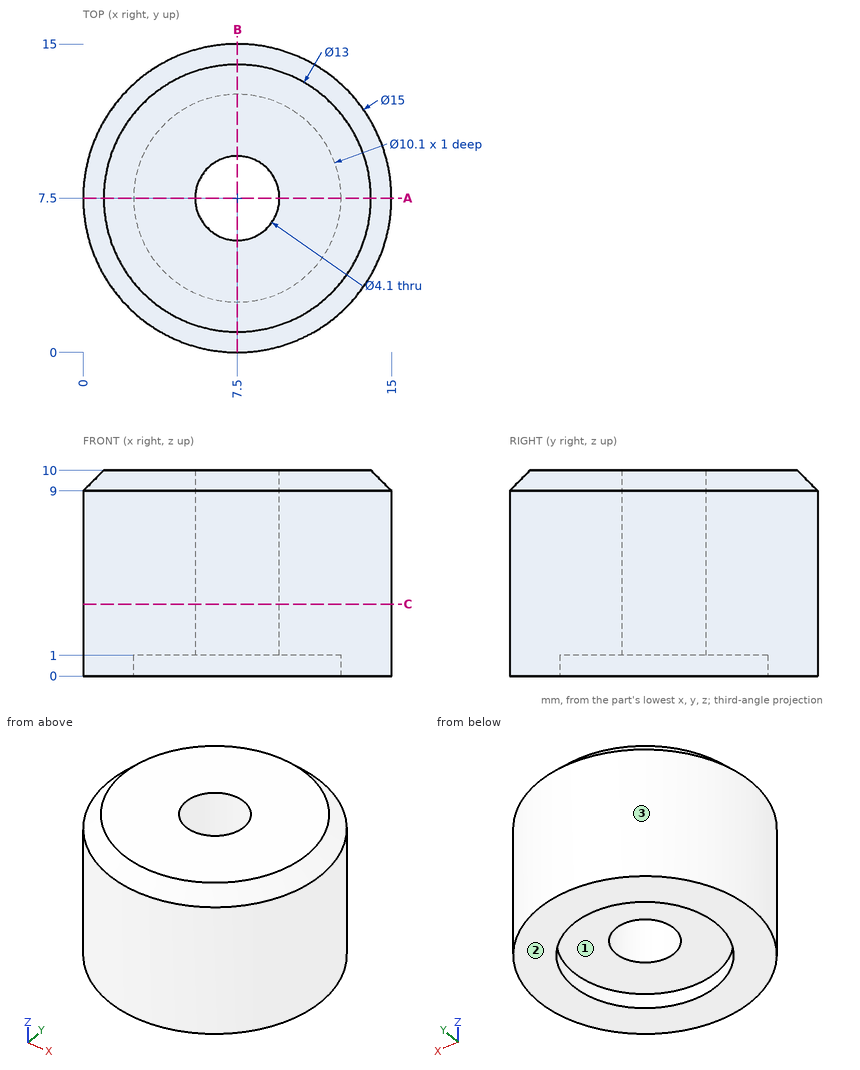
Print and shaded views of the part. All mm, measured from the part's lowest x, y and z. Coordinates: 2 decimals unless noted, no trailing zeros. Write each loop counter-clockwise with the first axis right and the second up, starting at its lowest first coordinate (ties: lowest second). Pieces come first, ordered by that corner, then holes.
(1) Two-plate mould, pull along X, no slides. Class the marked faces 1, 2 and 3: +X half, -X half, draft (parallel to the pull), parting line (faces both ways), or undercut.
(2) Cut at A-A, the plane y = 7.5. List the corners of the cut face in (x, z).
(3) Cut at C-C, the plane z = 3.5. List the corners of the cut face in (x, y), and give its area (3 significant figures).
(4) Drill centre lines: probe 1 along Y at (x, z) = (7.5, 8.25); probe 2 along Y at (x, z) = (7.5, 0.5); probe 3 along Z at (x, y) = (10.25, 5.75). Where is each one in solid material? Low to high.
(5) Flat gauge pins, fed straight in: pin 1 (2 mm diameter, centred on y = 6, z = 6, fed in from -X); pin 2 (5 mm diameter, centred on x = 9.5, y = 8.5, fed in from -Z). Where does each tip first touch, or does it go through?
Geometry says:
1. face 1: undercut
1. face 2: draft
1. face 3: parting line
2. outline: (0, 0) - (2.45, 0) - (2.45, 1) - (5.45, 1) - (5.45, 10) - (1, 10) - (0, 9) - close; (9.55, 1) - (12.55, 1) - (12.55, 0) - (15, 0) - (15, 9) - (14, 10) - (9.55, 10) - close
3. outline: circle Ø15 at (7.5, 7.5); hole circle Ø4.1 at (7.5, 7.5)
3. area: 164 mm2
4. probe 1: y = 0 to 5.45, 9.55 to 15
4. probe 2: y = 0 to 2.45, 12.55 to 15
4. probe 3: z = 1 to 10
5. pin 1: stops at x = 0.02
5. pin 2: stops at z = 1
